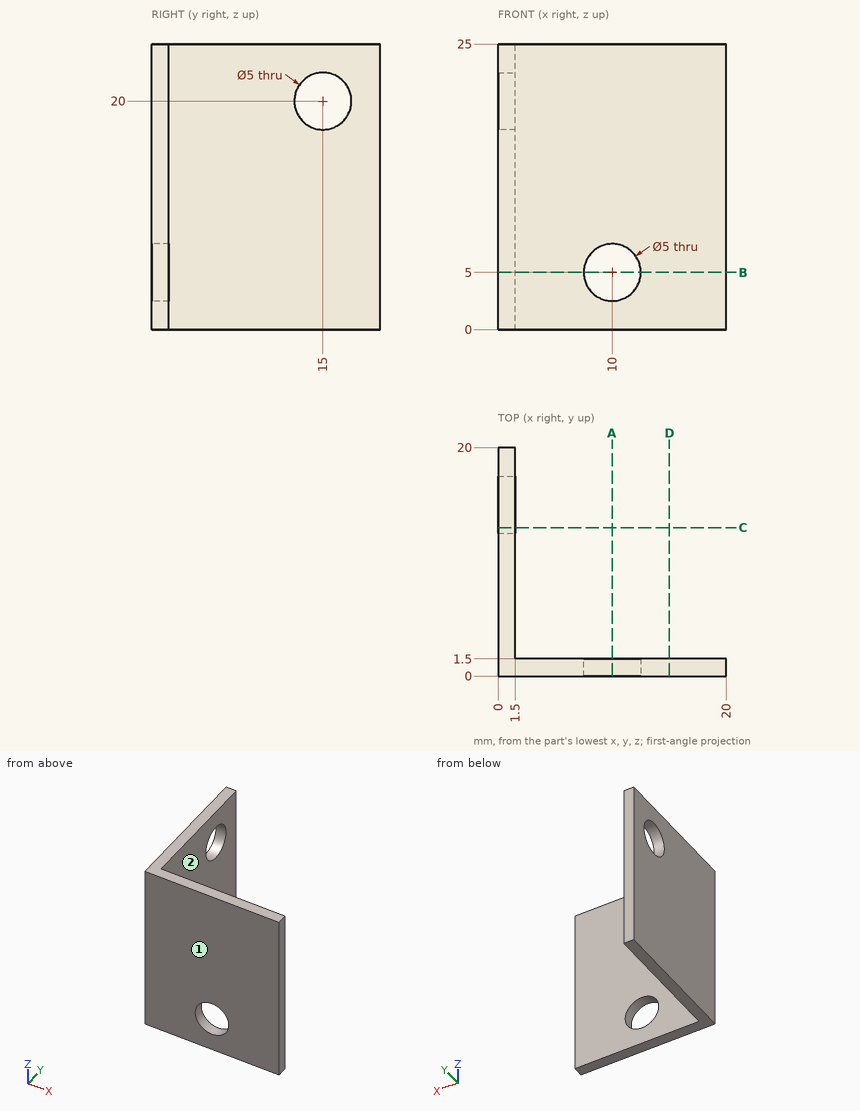
Could you check a few things on this drawing? It's one solid part, dimensions in mm from its lowest x, y, z. A direction names the side the tool comes from. Coordinates: 2 decimals unless noted, no trailing zeros. Order: outer loops, then holes, each group sorted by start corner. A loop starts at its lowest first (then second) coordinate and runs counter-clockwise, first axis right, second up. Notation, with made-up numbers: M 14,24.5 L 29,24.5 A17 ccw 29,29.5 Z; hole C 19.5,-19 d3. An arc over 180 degrees is marked long. Use a Markdown table: item, result. Add a question column.
Q1. I'm going to push flat-ended pins straight in: pin 1 (3 mm diameter, centred on y = 15, z = 20, fed in from +X); pin 2 (12 mm diameter, centred on y = 13, z = 17.5, fed in from +X); pin 3 (6 mm diameter, centred on x = 10, z = 5, fed in from +Y). Where does each tip first touch, or does it pass through?
Q2. I want a section at C-C on y = 13. List the corners of the cut face in (x, z) for me.
Q3. I want a section at A-A on x = 10. List the corners of the cut face in (y, z) for me.
Q4. I want a section at D-D on x = 15. List the corners of the cut face in (y, z) for me.
Q5. If I drill on L1, parallel to Z at x = 10, y = 0.95; L2, parallel to Y at x = 0.7, z = 20; L3, parallel to Y at x = 4.25, z = 18.5, over which ranges is the centre line in solid material (lowest first)?
Q6. Which directions (+Z, -Z, +X, -X, +Y, -Y) give clear straight access to the entire face, cutting with the end or side of a thin tool? Please do the marked faces 1 and 2.
Q7. I want a section at B-B on z = 5. List the corners of the cut face in (x, y) for me, then the cut area to 4 significant figures.
Checked values:
| question | item | result |
|---|---|---|
| 1 | pin 1 | through |
| 1 | pin 2 | x = 1.5 |
| 1 | pin 3 | y = 1.5 |
| 2 | outline | M 0,0 L 1.5,0 L 1.5,18.5 L 0,18.5 Z; M 0,21.5 L 1.5,21.5 L 1.5,25 L 0,25 Z |
| 3 | outline | M 0,0 L 1.5,0 L 1.5,2.5 L 0,2.5 Z; M 0,7.5 L 1.5,7.5 L 1.5,25 L 0,25 Z |
| 4 | outline | M 0,0 L 1.5,0 L 1.5,25 L 0,25 Z |
| 5 | L1 | 0 to 2.5, 7.5 to 25 |
| 5 | L2 | 0 to 12.5, 17.5 to 20 |
| 5 | L3 | 0 to 1.5 |
| 6 | face 1 | +Z, -Z, +X, -X, -Y |
| 6 | face 2 | +Z, -Z, +X, +Y |
| 7 | outline | M 0,0 L 7.5,0 L 7.5,1.5 L 1.5,1.5 L 1.5,20 L 0,20 Z; M 12.5,0 L 20,0 L 20,1.5 L 12.5,1.5 Z |
| 7 | area | 50.25 mm² |
